Answer from the drawing. Dimensions are ordinates in mm from the lowest x, y and z of the part. A direction names the side the tool comes from. Give positions to 0.01 mm unless a question says otherwise; leave off trailing zeros. Loops run counter-clockwise (first coordinate to the right, second up) from the corner with the lowest first, then second, coordinate; pieces in that order, holes last.
Item 1: Section C-C, the plane x = 6 is taken. Give the vertices of the cut face in (y, z) (1 decimal).
Item 2: Consider line 1 along Y through (x, z) = (59, 4) (1 decimal); line 2 along X through (y, z) = (14.5, 30.5) (1 decimal); line 3 along X through (y, z) = (23.75, 42). Determine where each line is inside the solid, lowest interval first.
Item 3: Section A-A, the plane z = 54 is taken. Give the vertices of the cut face in (x, y) (1 decimal), and give its area (3 significant figures).
Item 4: The mould has two halves that part along Y. Classify the marked faces 1, 2, 3 and 4: pulls with the +Y half, pulls with the -Y half, needs draft (parallel to the pull), parting line crosses it, or undercut.
Item 5: A tool of negligible diameter and unlimited length cuts with its end or side. For the marked faces 5 and 6, from which of +Z, -Z, +X, -X, +Y, -Y can it reach the whole face along a straight path? Write none if from no direction.
Item 6: Section B-B, the plane y = 21 is taken. Give the vertices of the cut face in (x, z) (1 decimal).
Item 7: Section D-D, the plane z = 38.1 is taken. Give the vertices of the cut face in (x, y) (1 decimal).
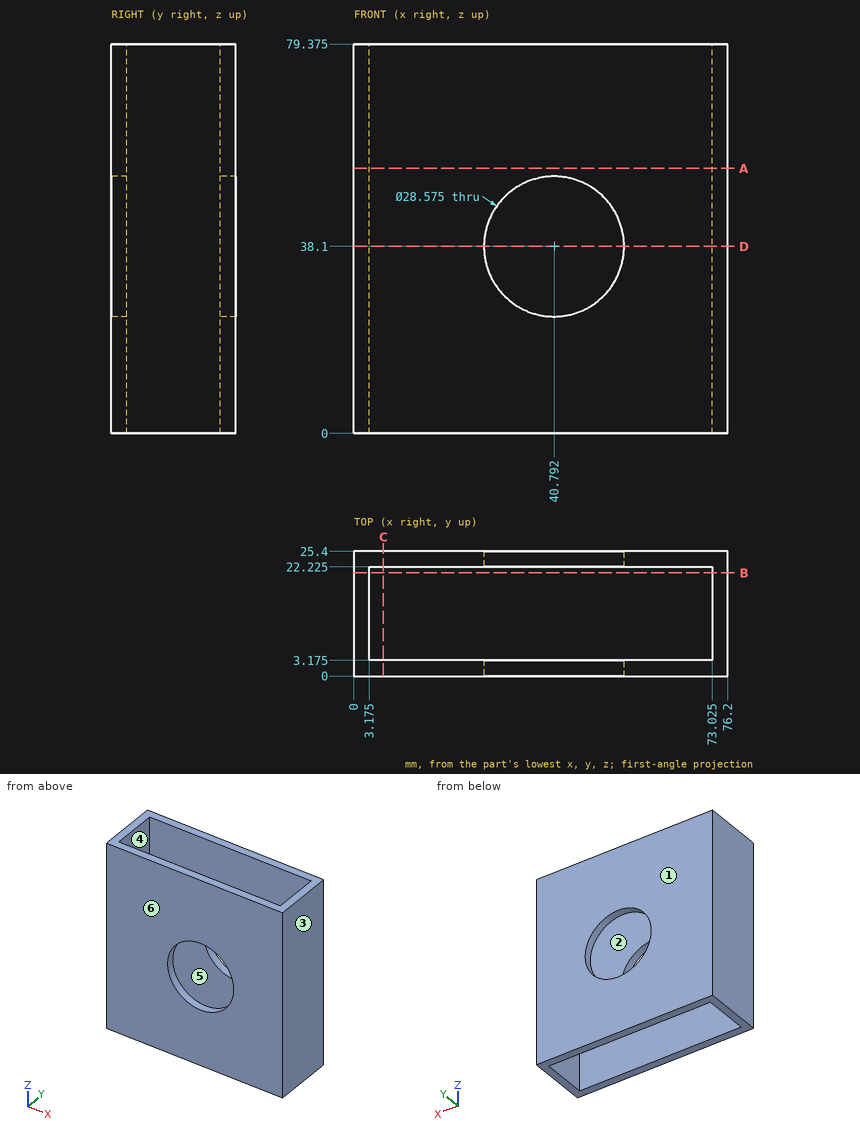
Worked answers:
1. outline: (0, 0) - (3.2, 0) - (3.2, 79.4) - (0, 79.4) - close; (22.2, 0) - (25.4, 0) - (25.4, 79.4) - (22.2, 79.4) - close
2. line 1: y = 0 to 3.2, 22.2 to 25.4
2. line 2: x = 0 to 3.2, 73 to 76.2
2. line 3: x = 0 to 27.05, 54.54 to 76.2
3. outline: (0, 0) - (76.2, 0) - (76.2, 25.4) - (0, 25.4) - close; hole (3.2, 3.2) - (73, 3.2) - (73, 22.2) - (3.2, 22.2) - close
3. area: 605 mm2
4. face 1: pulls with the +Y half
4. face 2: undercut
4. face 3: needs draft
4. face 4: undercut
5. face 5: +Z, -Z
5. face 6: +Z, -Z, +X, -X, -Y
6. outline: (0, 0) - (3.2, 0) - (3.2, 79.4) - (0, 79.4) - close; (73, 0) - (76.2, 0) - (76.2, 79.4) - (73, 79.4) - close
7. outline: (0, 0) - (26.5, 0) - (26.5, 3.2) - (3.2, 3.2) - (3.2, 22.2) - (26.5, 22.2) - (26.5, 25.4) - (0, 25.4) - close; (55.1, 0) - (76.2, 0) - (76.2, 25.4) - (55.1, 25.4) - (55.1, 22.2) - (73, 22.2) - (73, 3.2) - (55.1, 3.2) - close
